from build123d import *

# Parameters (mm, degrees)
F1_DEPTH = 50.8
F2_SIZE  = 2.54
F3_SIZE  = 2.54
F4_SIZE  = 2.54
F5_R     = 2.54
F6_R     = 2.54
F7_DEPTH = 25.4


with BuildPart() as f1:
    # F0 (on Top) → F1 (new body)
    with BuildSketch(Plane.XY):
        with BuildLine():
            Line((-25.396921, 0), (-11.509477, 0))
            ThreePointArc((-11.509477, 0), (-8.138429, 8.138429), (0, 11.509477))
            Line((0, 11.509477), (0, 12.709918))
            Line((0, 12.709918), (-18.907823, 12.709918))
            Line((-18.907823, 12.709918), (-18.907823, 9.544055))
            Line((-18.907823, 9.544055), (-21.449404, 9.544055))
            Line((-21.449404, 9.544055), (-21.449404, 12.709918))
            Line((-21.449404, 12.709918), (-25.396921, 12.709918))
            Line((-25.396921, 12.709918), (-25.396921, 0))
        make_face()
        with BuildLine():
            Line((0, 12.709918), (0, 11.509477))
            ThreePointArc((0, 11.509477), (8.138429, 8.138429), (11.509477, 0))
            Line((11.509477, 0), (25.405249, 0))
            Line((25.405249, 0), (25.405249, 12.709918))
            Line((25.405249, 12.709918), (21.477405, 12.709918))
            Line((21.477405, 12.709918), (21.477405, 9.544055))
            Line((21.477405, 9.544055), (18.936489, 9.544055))
            Line((18.936489, 9.544055), (18.936489, 12.709918))
            Line((18.936489, 12.709918), (0, 12.709918))
        make_face()
    extrude(amount=F1_DEPTH)

    # F2
    f2_edges = [f1.edges().sort_by_distance(p)[0] for p in [
        (21.477405, 12.709918, 25.4),
    ]]
    chamfer(f2_edges, length=F2_SIZE)

    # F3
    f3_edges = [f1.edges().sort_by_distance(p)[0] for p in [
        (-21.449404, 12.709918, 25.4),
        (18.936489, 12.709918, 25.4),
    ]]
    chamfer(f3_edges, length=F3_SIZE)

    # F4
    f4_edges = [f1.edges().sort_by_distance(p)[0] for p in [
        (-18.907823, 12.709918, 25.4),
    ]]
    chamfer(f4_edges, length=F4_SIZE)

    # F5
    f5_edges = [f1.edges().sort_by_distance(p)[0] for p in [
        (-11.509477, 0, 25.4),
        (11.509477, 0, 25.4),
    ]]
    fillet(f5_edges, radius=F5_R)

    # F6 (on face) → F7 (join)
    with BuildSketch(Plane(origin=(0, 12.709918, 0), x_dir=(-1, 0, 0), z_dir=(0, 1, 0))):
        with Locations((-13.342786, 41.559178)):
            Circle(F6_R)
        with Locations((13.342786, 41.559178)):
            Circle(F6_R)
        with Locations((13.342786, 7.999768)):
            Circle(F6_R)
        with Locations((-13.342786, 7.999768)):
            Circle(F6_R)
    extrude(amount=-F7_DEPTH)


solid = f1.part
Here's how the part is built. I have some questions about the finished solid (model axes, mm). A direction names the side the tool comes from. Give positions to 0.01 mm unless a question says otherwise; leave off trailing zeros. Order: outer loops, then holes, each group sorted by start corner. A loop starts at its lowest first (then second) coordinate and runs counter-clockwise, first axis right, second up. Notation, with made-up numbers: M 11,38.5 L 40,38.5 A20 ccw 40,51.5 Z; hole C 47.25,3.5 d3. An arc over 180 degrees is marked long. Answer as a JSON object with one key per item and string values. Group by question number.
1) Suppose I cut it at A-A, the plane y = 7.75. Write out the boundary of the cut face in (x, z), plus the area to 3 significant figures.
2) On a 3-axis mill with a long thin cutter (end or side, diameter ignored), from which of +Z, -Z, +X, -X, +Y, -Y can I reach the whole of each face in a straight line? I mean faces 4 (the cylindrical face through (-12.211, 0.573, 3.277)), 5 (the cylindrical face through (10.92, -6.09, 42.32)), 6 (the flat face through (-22.7, 11.42, 25.04)). Say none if no direction works.
3) Suppose I cut it at B-B, the plane z = 34.5. Write out the boundary of the cut face in (x, y).
4) Suppose I cut it at C-C, the plane y = 2.75. Write out the boundary of the cut face in (x, z).
5) Suppose I cut it at D-D, the plane y = -7.5. Write out the boundary of the cut face in (x, z), plus the area to 3 significant figures.
6) We'd pull the mould along X, two halves only. Please class faces 1 (the flat face through (13, -12.69, 42)), 2 (the cylindrical face through (-12.211, 0.573, 24.993)), 3 (the flat face through (25.405, 6, 25)): pulls with the +X half, pulls with the -X half, needs draft (parallel to the pull), parting line crosses it, or undercut.
7) Please list where these lines run through material, in increasing order: L1, parallel to X at y = -10.5, z = 8; L2, parallel to X at y = 4, z = 9.5; L3, parallel to Y at x = 15, z = 17.5. Write a range as [from, to].
8) I'm going to push flat-ended pins straight in: pin 1 Ø1.3 at (x, z) = (20, 37.5) entering from +Y; pin 2 Ø9.5 at (x, z) = (-17, 33) entering from -Y; pin 3 Ø3 at (x, z) = (-5, 30) entering from -Y; pin 4 Ø12 at (x, y) = (-4, 2) entering from -Z. Where does each tip first touch, or does it pass through?
Results found:
{
 "1": {"outline": "M -25.4,0 L -8.51,0 L -8.51,50.8 L -25.4,50.8 Z; M 8.51,0 L 25.41,0 L 25.41,50.8 L 8.51,50.8 Z", "area": "1,720 mm²"},
 "2": {"face 4": "-Z, -Y", "face 5": "-Y", "face 6": "+Z, -Z, +Y"},
 "3": {"outline": "M -25.4,0 L -13.82,0 A2.54 ccw -11.32,2.08 A11.51 cw 0,11.51 A11.51 cw 11.32,2.08 A2.54 ccw 13.82,0 L 25.41,0 L 25.41,12.71 L 24.02,12.71 L 21.48,10.17 L 21.48,9.54 L 18.94,9.54 L 18.94,10.17 L 16.4,12.71 L -16.37,12.71 L -18.91,10.17 L -18.91,9.54 L -21.45,9.54 L -21.45,10.17 L -23.99,12.71 L -25.4,12.71 Z"},
 "4": {"outline": "M -25.4,0 L -11.18,0 L -11.18,6.67 A2.54 ccw -11.18,9.33 L -11.18,40.23 A2.54 ccw -11.18,42.88 L -11.18,50.8 L -25.4,50.8 Z; M 11.18,0 L 25.41,0 L 25.41,50.8 L 11.18,50.8 L 11.18,42.88 A2.54 ccw 11.18,40.23 L 11.18,9.33 A2.54 ccw 11.18,6.67 Z"},
 "5": {"outline": "C -13.34,8 d5.08; C -13.34,41.56 d5.08; C 13.34,8 d5.08; C 13.34,41.56 d5.08", "area": "81.1 mm²"},
 "6": {"face 1": "needs draft", "face 2": "undercut", "face 3": "pulls with the +X half"},
 "7": {"L1": "[-15.88, -10.8], [10.8, 15.88]", "L2": "[-25.4, -10.79], [10.79, 25.41]", "L3": "[0, 12.71]"},
 "8": {"pin 1": "y = 9.54", "pin 2": "y = 0", "pin 3": "y = 9.5", "pin 4": "through"}
}
